Source: three-view drawing plus pictorial views. Frame: mm from the lowest corner of the part. A direction names the side the tool comes from. Coordinates: 2 decimals unless noted, no trailing zeros. Write each loop counter-clockwise with the first axis right and the second up, starting at its lowest first coordinate (ties: lowest second). Pieces come first, ordered by that corner, then holes. Notation, with made-up numbers: (1.5, -21) -> (34.5, -21) arc R31 ccw to (34.5, 15) -> close; hole circle Ø8 at (-2.5, 13.5). An arc over 180 degrees is marked (long way). Write item = value, one per line.
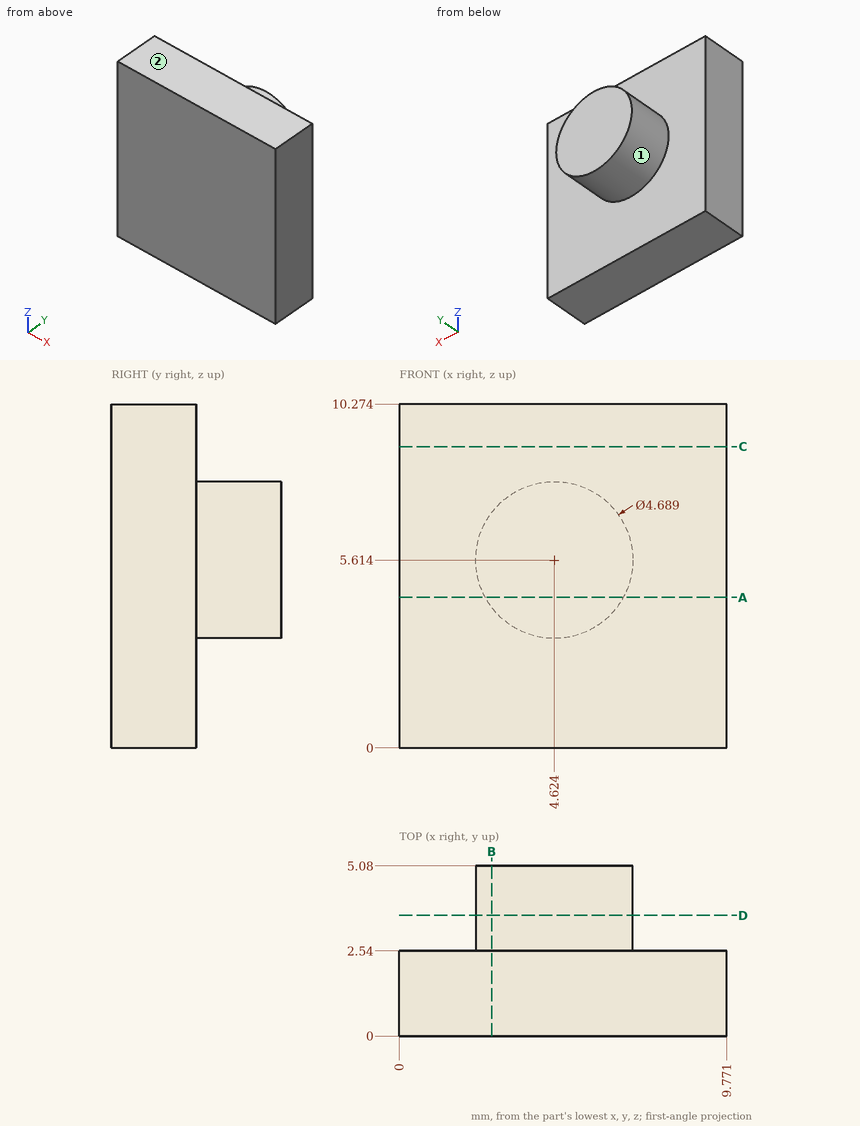
1) First-contact query: pin 1 Ø1.5 at (x, z) = (3.5, 2.5) entering from +Y. Flat tip, straight axial feed; report the tip coordinate or a pass-through.
Answer block:
pin_1 = 2.54
2) Cut plane B-B, the plane x = 2.75. Output: boundary loops of the cut face in (y, z) (1 decimal).
Answer block:
outline = (0, 0) -> (2.5, 0) -> (2.5, 4.2) -> (5.1, 4.2) -> (5.1, 7) -> (2.5, 7) -> (2.5, 10.3) -> (0, 10.3) -> close
3) Cut plane A-A, the plane z = 4.5. Output: boundary loops of the cut face in (x, y).
Answer block:
outline = (0, 0) -> (9.77, 0) -> (9.77, 2.54) -> (6.69, 2.54) -> (6.69, 5.08) -> (2.56, 5.08) -> (2.56, 2.54) -> (0, 2.54) -> close
4) Material intervals for probe 1 along Y at (x, z) = (6, 2.5); probe 2 along X at (y, z) = (4.6, 7.5) (1 decimal); probe 3 along Z at (x, y) = (3, 4.05) (1 decimal), sorted ascending. Write a range as [from, to].
Answer block:
probe_1 = [0, 2.54]
probe_2 = [3.2, 6]
probe_3 = [3.9, 7.3]
5) Cut plane C-C, the plane z = 9. Output: boundary loops of the cut face in (x, y).
Answer block:
outline = (0, 0) -> (9.77, 0) -> (9.77, 2.54) -> (0, 2.54) -> close
6) Reachability of the marked faces 1 and 2 from +Z, -Z, +X, -X, +Y, -Y: full face, straight path, thin tool, end or side. Return the list, or none.
Answer block:
face_1 = +Y
face_2 = +Z, +X, -X, +Y, -Y
7) Cut plane D-D, the plane y = 3.6. Output: boundary loops of the cut face in (x, z) (1 decimal), and give its area (3 significant figures).
Answer block:
outline = circle Ø4.7 at (4.6, 5.6)
area = 17.3 mm2
